Design review of the part built by this model. Coordinates are the model's own, in mm. Round coordinates to 2 decimals unless told otherwise and drop trailing zeros. Order: outer loops, then holes, each group sorted by start corner. A loop starts at its lowest first (then second) coordinate and runs counter-clockwise, first axis right, second up. Notation, with made-up numbers: (34.25, -36) - (74.25, -36) arc R3 cw to (74.25, -32) - close; hole circle Ø4 at (-24.5, 59.25). An arc over 180 degrees is marked (long way). Write item = value, one per line.
from build123d import *

# Parameters (mm, degrees)
SKETCH1_W                = 20
SKETCH1_H                = 20
BOSS_EXTRUDE1_DEPTH      = 228
FILLET1_R                = 1
CUT_EXTRUDE1_DEPTH       = 229.438175444
F_5_0_5_DIAMETER_HOLE1_D = 5
FILLET2_R                = 2
FILLET3_R                = 0.5
FILLET4_R                = 0.5
FILLET5_R                = 0.5


with BuildPart() as part:
    # Sketch1 → Boss-Extrude1 (new body)
    with BuildSketch(Plane(origin=(0, 0, 0), x_dir=(0, 0, -1), z_dir=(1, 0, 0))):
        Rectangle(SKETCH1_W, SKETCH1_H)
    extrude(amount=BOSS_EXTRUDE1_DEPTH)

    # Fillet1
    fillet1_edges = [part.edges().sort_by_distance(p)[0] for p in [
        (114, 10, 10),
        (114, 10, -10),
        (114, -10, -10),
        (114, -10, 10),
    ]]
    fillet(fillet1_edges, radius=FILLET1_R)

    # Sketch3 → Cut-Extrude1 (cut, through all)
    with BuildSketch(Plane.ZY):
        Polygon((-3.6, 10), (3.6, 10), (3.6, 9.5), (3.1, 9.5), (3.1, 8.2), (5.63, 8.2), (5.63, 6.619949494), (2.910050506, 3.9), (-2.910050506, 3.9), (-5.63, 6.619949494), (-5.63, 8.2), (-3.1, 8.2), (-3.1, 9.5), (-3.6, 9.5), align=None)
        Polygon((10, 3.6), (10, -3.6), (9.5, -3.6), (9.5, -3.1), (8.2, -3.1), (8.2, -5.63), (6.619949494, -5.63), (3.9, -2.910050506), (3.9, 2.910050506), (6.619949494, 5.63), (8.2, 5.63), (8.2, 3.1), (9.5, 3.1), (9.5, 3.6), align=None)
        Polygon((3.6, -10), (-3.6, -10), (-3.6, -9.5), (-3.1, -9.5), (-3.1, -8.2), (-5.63, -8.2), (-5.63, -6.619949494), (-2.910050506, -3.9), (2.910050506, -3.9), (5.63, -6.619949494), (5.63, -8.2), (3.1, -8.2), (3.1, -9.5), (3.6, -9.5), align=None)
        Polygon((-10, -3.6), (-10, 3.6), (-9.5, 3.6), (-9.5, 3.1), (-8.2, 3.1), (-8.2, 5.63), (-6.619949494, 5.63), (-3.9, 2.910050506), (-3.9, -2.910050506), (-6.619949494, -5.63), (-8.2, -5.63), (-8.2, -3.1), (-9.5, -3.1), (-9.5, -3.6), align=None)
    extrude(amount=-CUT_EXTRUDE1_DEPTH, mode=Mode.SUBTRACT)

    # Ø5.0 (5) Diameter Hole1 (through all)
    with Locations(Plane.ZY):
        with Locations((0, 0)):
            Hole(F_5_0_5_DIAMETER_HOLE1_D / 2)

    # Fillet2
    fillet2_edges = [part.edges().sort_by_distance(p)[0] for p in [
        (114, -3.9, -2.910050506),
        (114, -3.9, 2.910050506),
        (114, 2.910050506, -3.9),
        (114, -2.910050506, -3.9),
        (114, -2.910050506, 3.9),
        (114, 2.910050506, 3.9),
        (114, 3.9, 2.910050506),
        (114, 3.9, -2.910050506),
    ]]
    fillet(fillet2_edges, radius=FILLET2_R)

    # Fillet3
    fillet3_edges = [part.edges().sort_by_distance(p)[0] for p in [
        (114, 3.6, -10),
        (114, 3.1, -9.5),
        (114, 3.1, -8.2),
        (114, 5.63, -8.2),
        (114, 5.63, -6.619949494),
        (114, 3.6, 10),
        (114, 3.1, 9.5),
        (114, 3.1, 8.2),
        (114, 5.63, 8.2),
        (114, 5.63, 6.619949494),
        (114, 6.619949494, 5.63),
        (114, 8.2, 5.63),
        (114, 8.2, 3.1),
        (114, 9.5, 3.1),
        (114, 10, 3.6),
        (114, 9.5, -3.1),
        (114, 10, -3.6),
        (114, 8.2, -3.1),
        (114, 8.2, -5.63),
        (114, 6.619949494, -5.63),
    ]]
    fillet(fillet3_edges, radius=FILLET3_R - 0.0001)  # a hair under: the kernel refuses the full size

    # Fillet4
    fillet4_edges = [part.edges().sort_by_distance(p)[0] for p in [
        (114, -3.6, 10),
        (114, -3.1, 9.5),
        (114, -3.1, 8.2),
        (114, -5.63, 8.2),
        (114, -5.63, 6.619949494),
        (114, -6.619949494, 5.63),
        (114, -8.2, 5.63),
        (114, -8.2, 3.1),
        (114, -10, 3.6),
        (114, -9.5, 3.1),
        (114, -10, -3.6),
        (114, -9.5, -3.1),
        (114, -8.2, -3.1),
        (114, -8.2, -5.63),
        (114, -6.619949494, -5.63),
        (114, -5.63, -6.619949494),
        (114, -5.63, -8.2),
        (114, -3.1, -8.2),
        (114, -3.1, -9.5),
        (114, -3.6, -10),
    ]]
    fillet(fillet4_edges, radius=FILLET4_R - 0.0001)  # a hair under: the kernel refuses the full size

    # Fillet5
    fillet5_edges = [part.edges().sort_by_distance(p)[0] for p in [
        (114, 3.6, 9.5),
        (114, 9.5, 3.6),
        (114, 9.5, -3.6),
        (114, 3.6, -9.5),
        (114, -3.6, 9.5),
        (114, -9.5, 3.6),
        (114, -9.5, -3.6),
        (114, -3.6, -9.5),
    ]]
    fillet(fillet5_edges, radius=FILLET5_R)


solid = part.part
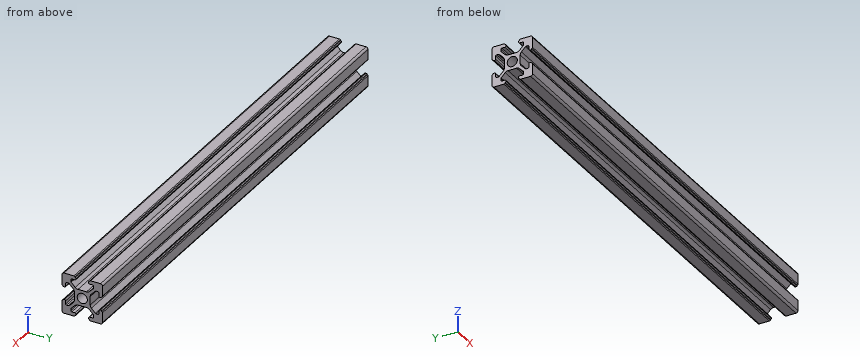
1) Clearance check with flat-ended pins moving along their axes: pin 1 Ø1.5 at (x, y) = (76.5, -0.5) entering from +Z; pin 2 Ø1.2 at (x, z) = (146.5, 0) entering from +Y. State where each tip first meets the part, or that it passes through.
Findings:
pin_1 = 3.9
pin_2 = 3.9
2) To check wall thickness, follow L1, parallel to Z at x = 37, y = -6.5; L2, parallel to Y at x = 110.5, z = 0; L3, parallel to Y at x = 173, z = -4.25. State the ranges of each line that lie inside material, in increasing order. Write a range as from..to.
Findings:
L1 = -10..-5.51, 5.51..10
L2 = -3.9..-2.5, 2.5..3.9
L3 = -10..-8.2, -5.24..-3.21, 3.21..5.24, 8.2..10
3) We need section A-A on y = 0. Write out the cut boundary in (x, z).
Findings:
outline = (0, -3.9) - (228, -3.9) - (228, -2.5) - (0, -2.5) - close; (0, 2.5) - (228, 2.5) - (228, 3.9) - (0, 3.9) - close
